Job drawing, mm, ordinate dimensions from the low corner. One solid piece. A direction names the side the tool comes from. Coordinates: 2 decimals unless noted, no trailing zeros. Loops run counter-clockwise (first coordinate to the right, second up) from the corner with the lowest first, then second, coordinate; pieces in that order, holes last. Notation, with made-up numbers: (-17.5, 38) - (40.5, 38) arc R23 ccw to (40.5, 66) - close; hole circle Ø3 at (49, 0). An arc over 180 degrees is marked (long way). One line per question, with ' | ' between items. Start each with the question number.
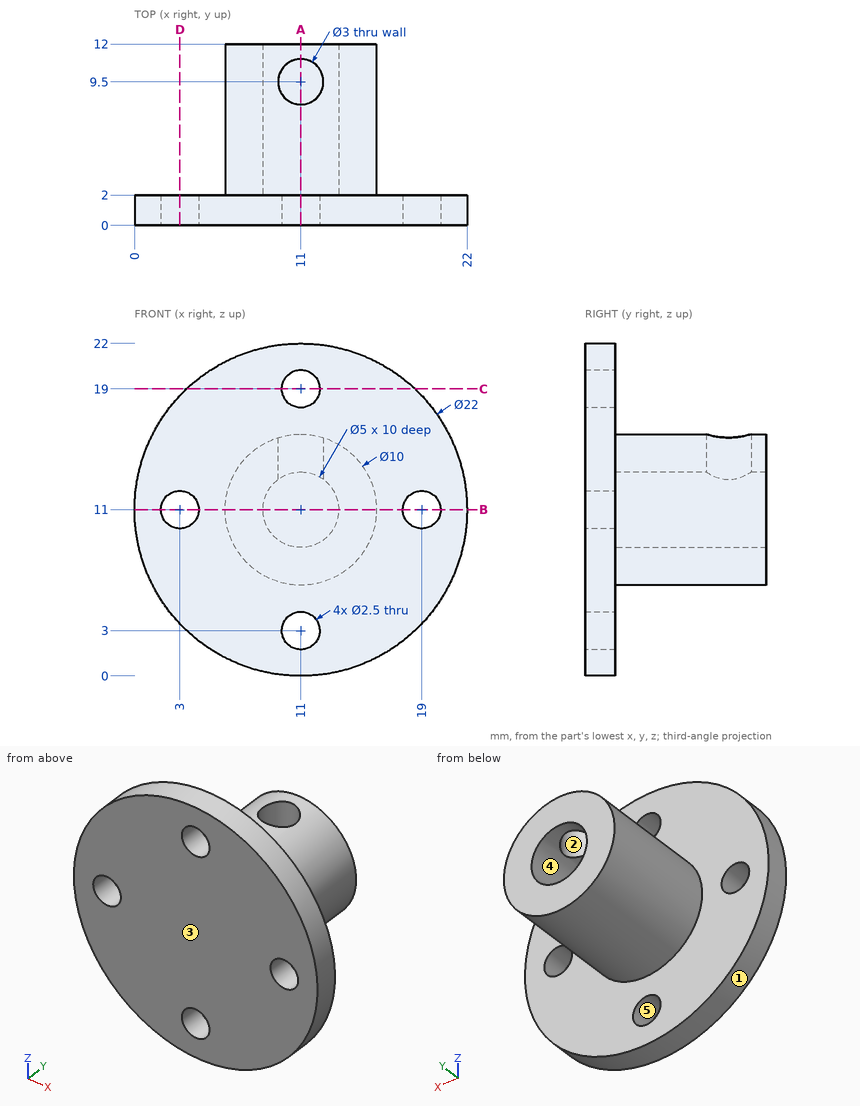
1) Band-saw the part on D-D on x = 3. List the corners of the cut face in (y, z), then the cut area to 3 significant figures.
2) Wall check: line 1 along X through (y, z) = (0.65, 11); line 2 along Y through (x, z) = (11, 14.15); line 3 along X through (y, z) = (6.75, 11). Give the ranges that are in metal, low to high. Write a range as [from, to].
3) Band-saw the part on C-C on z = 19. List the corners of the cut face in (x, y), then the cut area to 3 significant figures.
4) Pin check, flat tips, straight feed: pin 1 Ø1.5 at (x, z) = (19, 11) entering from +Y; pin 2 Ø1.5 at (x, z) = (11, 11) entering from +Y; pin 3 Ø5 at (x, y) = (11, 9.5) entering from +Z; pin 4 Ø2 at (x, y) = (9, 1) entering from -Z. Stop position of each tip, or through.
5) Band-saw the part on A-A on x = 11. List the corners of the cut face in (y, z), then the cut area to 3 significant figures.
6) Mould opens along X. For the marked faces 1, 2 and 3 say: +X half, -X half, draft (parallel to the pull), parting line (faces both ways), or undercut.
7) Tool access for the marked faces 4 and 5: list every direction of +Z, -Z, +X, -X, +Y, -Y with a clear straight run to the whole face (end or side of a thin tool).
8) Band-saw the part on B-B on z = 11. List the corners of the cut face in (x, y), then the cut area to 3 significant figures.
Values found:
1) outline: (0, 3.45) - (2, 3.45) - (2, 9.75) - (0, 9.75) - close; (0, 12.25) - (2, 12.25) - (2, 18.55) - (0, 18.55) - close | area: 25.2 mm²
2) line 1: [0, 1.75], [4.25, 17.75], [20.25, 22] | line 2: [0, 8], [11, 12] | line 3: [6, 8.5], [13.5, 16]
3) outline: (3.45, 0) - (9.75, 0) - (9.75, 2) - (3.45, 2) - close; (12.25, 0) - (18.55, 0) - (18.55, 2) - (12.25, 2) - close | area: 25.2 mm²
4) pin 1: through | pin 2: y = 2 | pin 3: z = 16 | pin 4: z = 0.05
5) outline: (0, 0) - (2, 0) - (2, 1.75) - (0, 1.75) - close; (0, 4.25) - (2, 4.25) - (2, 6) - (12, 6) - (12, 8.5) - (2, 8.5) - (2, 13.5) - (8, 13.5) - (8, 16) - (2, 16) - (2, 17.75) - (0, 17.75) - close; (0, 20.25) - (2, 20.25) - (2, 22) - (0, 22) - close; (11, 13.5) - (12, 13.5) - (12, 16) - (11, 16) - close | area: 76.5 mm²
6) face 1: parting line | face 2: undercut | face 3: draft
7) face 4: +Y | face 5: +Y, -Y
8) outline: (0, 0) - (1.75, 0) - (1.75, 2) - (0, 2) - close; (4.25, 0) - (17.75, 0) - (17.75, 2) - (16, 2) - (16, 12) - (13.5, 12) - (13.5, 2) - (8.5, 2) - (8.5, 12) - (6, 12) - (6, 2) - (4.25, 2) - close; (20.25, 0) - (22, 0) - (22, 2) - (20.25, 2) - close | area: 84.0 mm²
